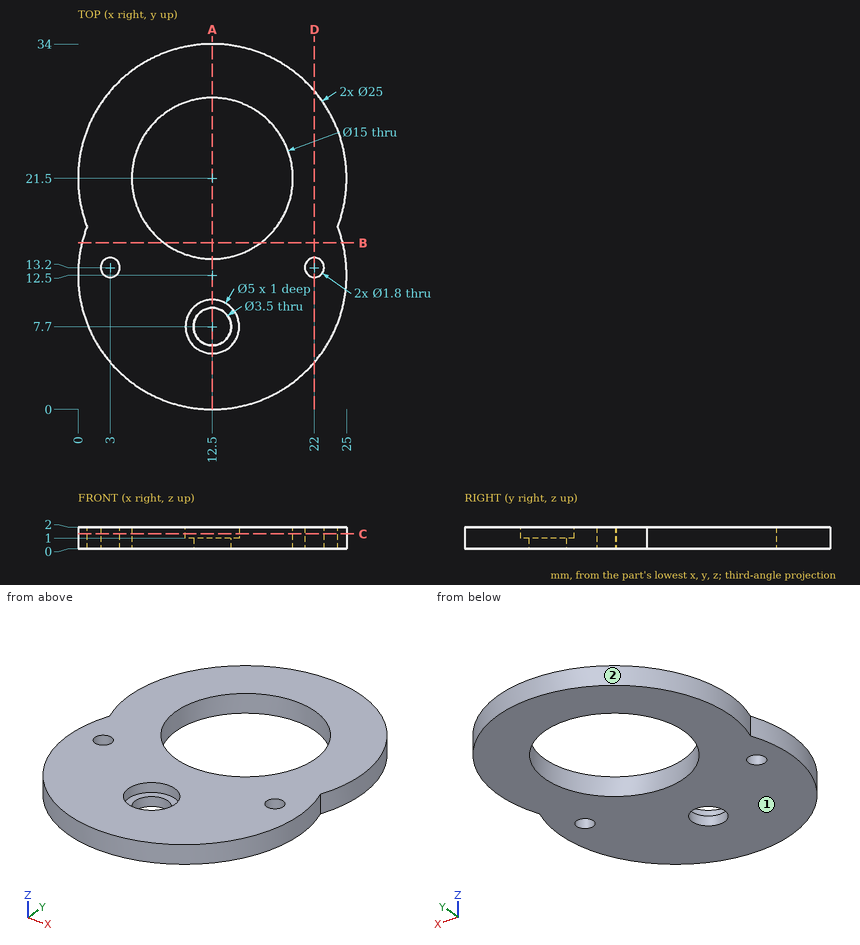
Geometry: see drawing. Coordinates: mm, zero at the bounding-box minimum. Coordinates: 2 decimals unless noted, no trailing zeros. Loops run counter-clockwise (first coordinate to the right, second up) from the corner with the lowest first, then second, coordinate; pieces in that order, holes last. Notation, with made-up numbers: M -33.5,65.25 L 5.5,65.25 A27 ccw 5.5,98.25 Z; hole C -1,-12.75 d3. An arc over 180 degrees is marked long. Put each result on its own line as item: value. Start each with the question number.
1) Cut plane A-A on x = 12.5. Return the cut outline in (y, z).
2) Contact query for flat-ended pins moving along their axis: pin 1 Ø4 at (x, y) = (13.5, 7) entering from +Z; pin 2 Ø4 at (x, y) = (12.5, 7.7) entering from +Z; pin 3 Ø1.6 at (x, y) = (22, 13.2) entering from -Z; pin 4 Ø1 at (y, z) = (16, 0.5) entering from -X. Output: stop coordinate, or through.
3) Cut plane C-C on z = 1.4. Return the cut outline in (x, y).
4) Cut plane D-D on x = 22. Return the cut outline in (y, z), then the cut area to 3 significant figures.
5) Pull-direction query (Y, two-part tool) for the marked faces 1 and 2; classes: pulls with the +Y half, pulls with the -Y half, needs draft (parallel to the pull), parting line crosses it, or undercut.
6) Ray query, L1, parallel to Y at x = 12, z = 1.1; L2, parallel to X at y = 28, z = 0.75; L3, parallel to Y at x = 3, z = 0.95. Return the intervals inside material, ascending. Write a range as from..to.
7) Cut plane B-B on y = 15.5. Return the cut outline in (x, z), then the cut area to 3 significant figures.
The answers:
1. outline: M 0,0 L 5.95,0 L 5.95,1 L 5.2,1 L 5.2,2 L 0,2 Z; M 9.45,0 L 14,0 L 14,2 L 10.2,2 L 10.2,1 L 9.45,1 Z; M 29,0 L 34,0 L 34,2 L 29,2 Z
2. pin 1: stops at z = 2
2. pin 2: stops at z = 1
2. pin 3: passes through
2. pin 4: stops at x = 0.37
3. outline: M 0.84,17 A12.5 ccw long 24.16,17 A12.5 ccw long Z; hole C 3,13.2 d1.8; hole C 12.5,21.5 d15; hole C 12.5,7.7 d5; hole C 22,13.2 d1.8
4. outline: M 4.38,0 L 12.3,0 L 12.3,2 L 4.38,2 Z; M 14.1,0 L 29.62,0 L 29.62,2 L 14.1,2 Z
4. area: 46.9 mm²
5. face 1: needs draft
5. face 2: undercut
6. L1: y = 0.01..5.25, 10.15..14.02, 28.98..33.99
6. L2: x = 1.82..8.76, 16.24..23.18
6. L3: y = 4.38..12.3, 14.1..29.62
7. outline: M 0.37,0 L 8,0 L 8,2 L 0.37,2 Z; M 17,0 L 24.63,0 L 24.63,2 L 17,2 Z
7. area: 30.5 mm²
